The model under review builds one solid part; all positions refer to its coordinate system, in mm. Coordinates: 2 decimals unless noted, no trailing zeros. Order: outer loops, then holes, each group sorted by start corner. A loop starts at its lowest first (then second) coordinate and runs counter-clockwise, first axis right, second up. Notation, with made-up numbers: (6, 35.5) -> (37, 35.5) arc R10 cw to (37, 45.5) -> close; hole circle Ø4 at (9, -26). An arc over 180 degrees is marked (long way). Use CSV: the item, a comma, the result in double quotes. Start each with the question number.
```python
from build123d import *

# Parameters (mm, degrees)
SKETCH1_W                      = 222.5
SKETCH1_H                      = 80
BOSS_EXTRUDE1_DEPTH            = 6.35
CUT_EXTRUDE1_DEPTH             = 119.392926309
CUT_EXTRUDE2_DEPTH             = 119.392926309
M5X0_8_TAPPED_HOLE1_AT_2_COUNT = 2
M5X0_8_TAPPED_HOLE1_AT_2_PITCH = 15
M5X0_8_TAPPED_HOLE1_AT_3_COUNT = 2
M5X0_8_TAPPED_HOLE1_AT_3_PITCH = 50
M5X0_8_TAPPED_HOLE1_AT_4_COUNT = 2
M5X0_8_TAPPED_HOLE1_AT_4_PITCH = 35
FILLET1_R                      = 7


with BuildPart() as part:
    # Sketch1 → Boss-Extrude1 (new body)
    with BuildSketch(Plane.XY):
        Rectangle(SKETCH1_W, SKETCH1_H)
    extrude(amount=BOSS_EXTRUDE1_DEPTH)

    # Sketch2 → Cut-Extrude1 (cut, through all)
    with BuildSketch(Plane.XY.offset(6.35)):
        Polygon((111.25, -40), (0, 0.491688562), (-111.25, -40), align=None)
    extrude(amount=-CUT_EXTRUDE1_DEPTH, mode=Mode.SUBTRACT)

    # Sketch3 → Cut-Extrude2 (cut, through all)
    with BuildSketch(Plane.XY.offset(6.35)):
        Polygon((-99.25, 33), (-99.25, -22.862223919), (-6, 11.078000426), (-6, 33), align=None)
    cut_extrude2 = extrude(amount=-CUT_EXTRUDE2_DEPTH, mode=Mode.SUBTRACT)

    # Sketch4 → M5x0.8 Tapped Hole1 (revolve, cut)
    with BuildSketch(Plane(origin=(-104.9, -25, 0), x_dir=(0, 1, 0), z_dir=(1, 0, 0))):
        Polygon((0, 0), (0, 13.6618073), (2.1, 12.4), (2.1, 0), align=None)
    m5x0_8_tapped_hole1 = revolve(axis=Axis((-104.9, -25, -6.35), (0, 0, 1)), mode=Mode.SUBTRACT)

    # M5x0.8 Tapped Hole1 at 2: M5x0.8 Tapped Hole1 ×2
    with Locations(*[(0, i * M5X0_8_TAPPED_HOLE1_AT_2_PITCH, 0) for i in range(1, M5X0_8_TAPPED_HOLE1_AT_2_COUNT)]):
        add(m5x0_8_tapped_hole1, mode=Mode.SUBTRACT)

    # M5x0.8 Tapped Hole1 at 3: M5x0.8 Tapped Hole1 ×2
    with Locations(*[(0, i * M5X0_8_TAPPED_HOLE1_AT_3_PITCH, 0) for i in range(1, M5X0_8_TAPPED_HOLE1_AT_3_COUNT)]):
        add(m5x0_8_tapped_hole1, mode=Mode.SUBTRACT)

    # M5x0.8 Tapped Hole1 at 4: M5x0.8 Tapped Hole1 ×2
    with Locations(*[(0, i * M5X0_8_TAPPED_HOLE1_AT_4_PITCH, 0) for i in range(1, M5X0_8_TAPPED_HOLE1_AT_4_COUNT)]):
        add(m5x0_8_tapped_hole1, mode=Mode.SUBTRACT)

    # Mirror1: Cut-Extrude2, M5x0.8 Tapped Hole1 across plane
    add(cut_extrude2.mirror(Plane(origin=(0, 0, 0), x_dir=(0, 0, 1), z_dir=(1, 0, 0))), mode=Mode.SUBTRACT)
    add(m5x0_8_tapped_hole1.mirror(Plane(origin=(0, 0, 0), x_dir=(0, 0, 1), z_dir=(1, 0, 0))), mode=Mode.SUBTRACT)

    # Mirror1 copy 1 sketch → Mirror1 copy 1 (revolve, cut)
    with BuildSketch(Plane(origin=(104.9, -10, 0), x_dir=(0, 1, 0), z_dir=(-1, 0, 0))):
        Polygon((0, 0), (0, -13.6618073), (2.1, -12.4), (2.1, 0), align=None)
    revolve(axis=Axis((104.9, -10, -6.35), (0, 0, -1)), mode=Mode.SUBTRACT)

    # Mirror1 copy 2 sketch → Mirror1 copy 2 (revolve, cut)
    with BuildSketch(Plane(origin=(104.9, 25, 0), x_dir=(0, 1, 0), z_dir=(-1, 0, 0))):
        Polygon((0, 0), (0, -13.6618073), (2.1, -12.4), (2.1, 0), align=None)
    revolve(axis=Axis((104.9, 25, -6.35), (0, 0, -1)), mode=Mode.SUBTRACT)

    # Mirror1 copy 3 sketch → Mirror1 copy 3 (revolve, cut)
    with BuildSketch(Plane(origin=(104.9, 10, 0), x_dir=(0, 1, 0), z_dir=(-1, 0, 0))):
        Polygon((0, 0), (0, -13.6618073), (2.1, -12.4), (2.1, 0), align=None)
    revolve(axis=Axis((104.9, 10, -6.35), (0, 0, -1)), mode=Mode.SUBTRACT)

    # Fillet1
    fillet1_edges = [part.edges().sort_by_distance(p)[0] for p in [
        (0, 0.491688562, 3.175),
        (-99.25, 33, 3.175),
        (-6, 33, 3.175),
        (-6, 11.078000426, 3.175),
        (-99.25, -22.862223919, 3.175),
        (6, 33, 3.175),
        (99.25, 33, 3.175),
        (99.25, -22.862223919, 3.175),
        (6, 11.078000426, 3.175),
        (111.25, -40, 3.175),
        (-111.25, -40, 3.175),
        (-111.25, 40, 3.175),
        (111.25, 40, 3.175),
    ]]
    fillet(fillet1_edges, radius=FILLET1_R)


solid = part.part
```
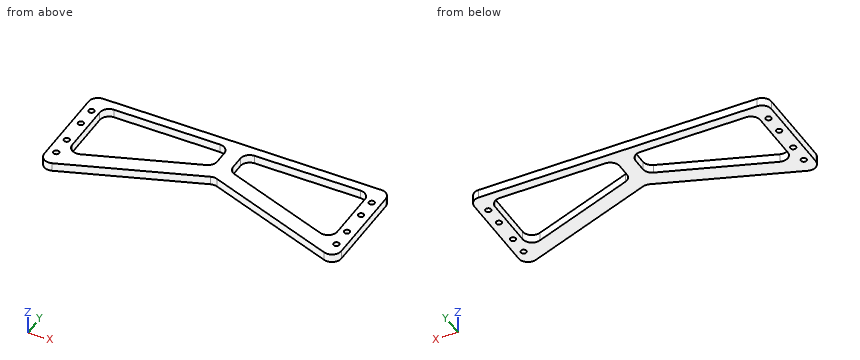
Q1. Add section C-C, the plane x = -57. State the section outline as (y, z) points.
Q2. Add section B-B, the plane z = 2. State how many separate pieces and enclosed holes the cut face has, then the cut area to 3 significant figures.
Q3. Clearance check with flat-ended pins moving along their axes: pin 1 Ø3 at (x, y) = (-66, -7.5) entering from +Z; pin 2 Ø5 at (x, y) = (-104.9, 10) entering from +Z; pin 3 Ø1 at (x, z) = (-49, 5.5) entering from -Y; pin 4 Ø3 at (x, z) = (35, 3) entering from -Y. State where each tip first meets the part, or that it passes through.
Q4. Add section A-A, the plane y = -25. State the section outline as (x, z) points.
Q5. Add section D-D, the plane y = 5.5. State the section outline as (x, z) points, then the cut area to 3 significant figures.
Q6. To check wall thickness, follow probe 1 along X at (y, z) = (18.5, 2.75); probe 2 along X at (y, z) = (25, 4.75); probe 3 along Y at (x, z) = (-104.9, 2). State the ranges of each line that lie inside material, in increasing order.
Answer block:
1,outline,"(-20.25, 0) -> (-7.48, 0) -> (-7.48, 6.35) -> (-20.25, 6.35) -> close; (33, 0) -> (40, 0) -> (40, 6.35) -> (33, 6.35) -> close"
2,separate pieces,"1"
2,enclosed holes,"10"
2,area,"5,960 mm²"
3,pin 1,"passes through"
3,pin 2,"stops at z = 6.35"
3,pin 3,"stops at y = -17.52"
3,pin 4,"stops at y = -12.79"
4,outline,"(-111.25, 0) -> (-107, 0) -> (-107, 6.35) -> (-111.25, 6.35) -> close; (-102.8, 0) -> (-70.04, 0) -> (-70.04, 6.35) -> (-102.8, 6.35) -> close; (70.04, 0) -> (102.8, 0) -> (102.8, 6.35) -> (70.04, 6.35) -> close; (107, 0) -> (111.25, 0) -> (111.25, 6.35) -> (107, 6.35) -> close"
5,outline,"(-111.25, 0) -> (-99.25, 0) -> (-99.25, 6.35) -> (-111.25, 6.35) -> close; (-21.33, 0) -> (21.33, 0) -> (21.33, 6.35) -> (-21.33, 6.35) -> close; (99.25, 0) -> (111.25, 0) -> (111.25, 6.35) -> (99.25, 6.35) -> close"
5,area,"423 mm²"
6,probe 1,"x = -111.25 to -99.25, -6 to 6, 99.25 to 111.25"
6,probe 2,"x = -111.25 to -107, -102.8 to -99.25, -6 to 6, 99.25 to 102.8, 107 to 111.25"
6,probe 3,"y = -36.97 to -27.1, -22.9 to -12.1, -7.9 to 7.9, 12.1 to 22.9, 27.1 to 39.97"
